Autodesk Inventor part; units mm, degrees
ref_plane "YZ Plane" through (0, 0, 0) normal (1, 0, 0) x (0, 1, 0)
ref_plane "XZ Plane" through (0, 0, 0) normal (0, 1, 0) x (-1, 0, 0)
ref_plane "XY Plane" through (0, 0, 0) normal (0, 0, 1) x (1, 0, 0)
sketch "Sketch1" plane through (0, 0, 0) normal (0, 0, 1) x (1, 0, 0)
  line L0 (-7.5633, 0) -> (-3.7816, 6.55)
  line L1 (-3.7816, 6.55) -> (3.7816, 6.55)
  line L2 (3.7816, 6.55) -> (7.5633, 0)
  line L3 (7.5633, 0) -> (3.7816, -6.55)
  line L4 (3.7816, -6.55) -> (-3.7816, -6.55)
  line L5 (-3.7816, -6.55) -> (-7.5633, 0)
  circle A0 centre (0, 0) radius 9
  circle A1 centre (0, 0) radius 2.45
  point P0 (0, -6.55)
  point P1 (0, 6.55)
  dimension "d0" = 13.1
  dimension "d1" = 18
  dimension "d2" = 4.9
extrude "Extrusion1" add sketch "Sketch1" along normal blind 8 contours A0
extrude "Extrusion2" add sketch "Sketch1" against normal blind 17.25 contours L0 L1 L2 L3 L4 L5 | A0
sketch "Sketch2" plane through (0, 0, -17.25) normal (0, 0, -1) x (-1, 0, 0)
  circle A0 centre (0, 0) radius 5
  dimension "d7" = 10
extrude "Extrusion3" cut sketch "Sketch2" against normal blind 12.75
properties part number "End Shaft Spacers"
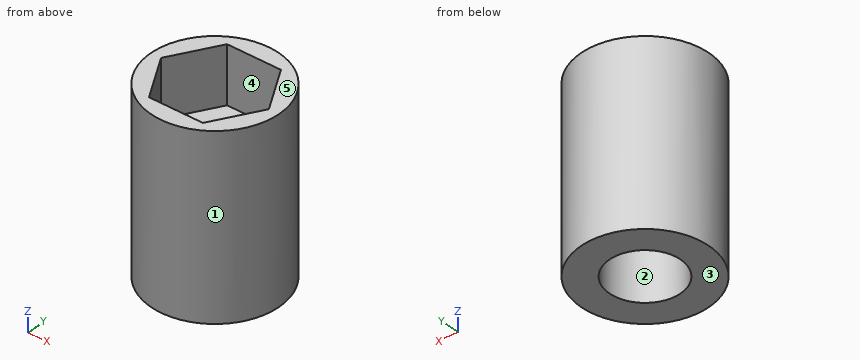
The listing builds one solid part. Answer for the finished solid, in the listing's coordinates (mm). Face numbers are marked on the shaded views. A direction names the side the tool comes from. Give positions to 0.01 mm unless a question says otherwise; leave off trailing zeros. Order: outer loops, then holes, each group sorted by start corner. A loop starts at its lowest first (then second) coordinate and runs counter-clockwise, first axis right, second up.
Item 1: Which of the six approach directions +Z, -Z, +X, -X, +Y, -Y give full straight-line access (tool end or side, diameter ignored) to the marked faces 4 and 5?
From the geometry:
face 4: +Z
face 5: +Z, +X, -X, +Y, -Y
Item 2: The part is cut by section A-A, the plane x = 0. Give the vertices of the cut face in (y, z), and give its area (3 significant figures).
From the geometry:
outline: (-9, -17.25) - (-5, -17.25) - (-5, -4.5) - (-2.45, -4.5) - (-2.45, 0) - (-6.55, 0) - (-6.55, 8) - (-9, 8) - close; (2.45, -4.5) - (5, -4.5) - (5, -17.25) - (9, -17.25) - (9, 8) - (6.55, 8) - (6.55, 0) - (2.45, 0) - close
area: 200 mm2
Item 3: Find the intervals of material crossed by probe 1 along Y at (x, z) = (0, -12.25); probe 2 along X at (y, z) = (-0.25, -10.25); probe 3 along Y at (x, z) = (0, -1.9), in increasing order.
From the geometry:
probe 1: y = -9 to -5, 5 to 9
probe 2: x = -9 to -4.99, 4.99 to 9
probe 3: y = -9 to -2.45, 2.45 to 9
Item 4: The part is cut by section D-D, the plane y = 6.25. Give the vertices of the cut face in (x, z), and give its area (3 significant figures).
From the geometry:
outline: (-6.48, -17.25) - (6.48, -17.25) - (6.48, 8) - (3.95, 8) - (3.95, 0) - (-3.95, 0) - (-3.95, 8) - (-6.48, 8) - close
area: 264 mm2
Item 5: For a pull along Y with two mould halves and no side action, classify the marked faces 1, 2 and 3 as pulls with the +Y half, pulls with the -Y half, needs draft (parallel to the pull), parting line crosses it, or undercut.
From the geometry:
face 1: parting line crosses it
face 2: undercut
face 3: needs draft
Item 6: The part is cut by section C-C, the plane y = 1.25. Give the vertices of the cut face in (x, z).
From the geometry:
outline: (-8.91, -17.25) - (-4.84, -17.25) - (-4.84, -4.5) - (-2.11, -4.5) - (-2.11, 0) - (-6.84, 0) - (-6.84, 8) - (-8.91, 8) - close; (2.11, -4.5) - (4.84, -4.5) - (4.84, -17.25) - (8.91, -17.25) - (8.91, 8) - (6.84, 8) - (6.84, 0) - (2.11, 0) - close
Item 7: The part is cut by section B-B, the plane z = 5.5. Give the vertices of the cut face in (x, y), and give its area (3 significant figures).
From the geometry:
outline: circle Ø18 at (0, 0); hole (-7.56, 0) - (-3.78, -6.55) - (3.78, -6.55) - (7.56, 0) - (3.78, 6.55) - (-3.78, 6.55) - close
area: 106 mm2
Item 8: Given pin 1 Ø3 at (y, z) = (-3.5, -7.5) entering from -X; pin 2 Ø3 at (y, z) = (-5, 4) entering from +X; pin 3 Ø3 at (x, y) = (-0.5, 1) entering from -Z; pin 4 Ø3 at (x, y) = (0, 0) entering from -Z, each flat-ended and moving along its own axis, determine where each tip first touches the part or whether it passes through.
From the geometry:
pin 1: stops at x = -8.77
pin 2: stops at x = 8.29
pin 3: stops at z = -4.5
pin 4: passes through
